Geometry: see drawing. Coordinates: mm, zero at the bounding-box minimum. Give positions to 0.01 mm unless a question says otherwise; leave off trailing zeros. Write each loop counter-clockwise with the first axis right and the second up, starting at its lowest first coordinate (ties: lowest second). Pieces come first, ordered by that corner, then holes. Notation, with made-up numbers: M 69.25,10 L 79.25,10 A13 cw 79.25,29 Z; hole C 23,-19 d6. An arc over 180 degrees is marked long. Use CSV: the item, a comma, the result in double quotes. Start each with the question number.
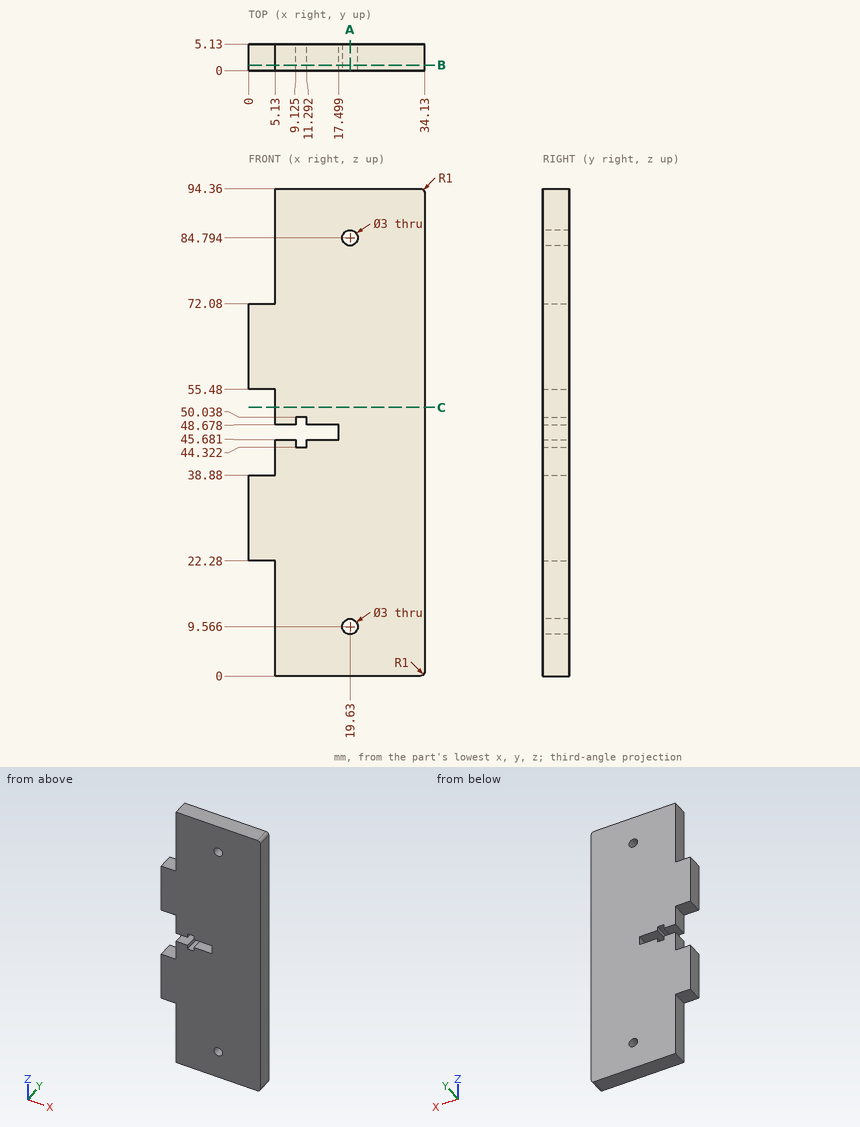
1. Section C-C on z = 52. Return loops of the section in (x, y).
2. Line query: probe 1 along Z at (x, y) = (19.63, 2.75) (1 decimal); probe 2 along Z at (x, y) = (15, 1.05); probe 3 along Z at (x, y) = (20, 1.7). Output: solid intervals per line, ascending.
3. Section A-A on x = 19.63. Return loops of the section in (y, z) (1 decimal).
4. Section B-B on y = 1.05. Return loops of the section in (x, z) (1 decimal).
5. First-contact query: pin 1 (2.5 mm diameter, centred on y = 2.5, z = 53, fed in from -X); pin 2 (2.5 mm diameter, centred on x = 3, y = 3.5, fed in from -Z). Flat tips, straight axial feed; report the tip coordinate or a pass-through.
Resolved:
1,outline,"M 5.13,0 L 34.13,0 L 34.13,5.13 L 5.13,5.13 Z"
2,probe 1,"z = 0 to 8.1, 11.1 to 83.3, 86.3 to 94.4"
2,probe 2,"z = 0 to 45.68, 48.68 to 94.36"
2,probe 3,"z = 0 to 8.11, 11.02 to 83.34, 86.25 to 94.36"
3,outline,"M 0,0 L 5.1,0 L 5.1,8.1 L 0,8.1 Z; M 0,11.1 L 5.1,11.1 L 5.1,83.3 L 0,83.3 Z; M 0,86.3 L 5.1,86.3 L 5.1,94.4 L 0,94.4 Z"
4,outline,"M 0,22.3 L 5.1,22.3 L 5.1,0 L 33.1,0 A1 ccw 34.1,1 L 34.1,93.4 A1 ccw 33.1,94.4 L 5.1,94.4 L 5.1,72.1 L 0,72.1 L 0,55.5 L 5.1,55.5 L 5.1,48.7 L 9.1,48.7 L 9.1,50 L 11.3,50 L 11.3,48.7 L 17.5,48.7 L 17.5,45.7 L 11.3,45.7 L 11.3,44.3 L 9.1,44.3 L 9.1,45.7 L 5.1,45.7 L 5.1,38.9 L 0,38.9 Z; hole C 19.6,9.6 d3; hole C 19.6,84.8 d3"
5,pin 1,"stops at x = 5.13"
5,pin 2,"stops at z = 22.28"
